Here's how the part is built. I have some questions about the finished solid (model axes, mm). Round coordinates to 2 decimals unless told otherwise and drop trailing zeros. Write each loop counter-clockwise with the first axis right and the second up, starting at its lowest first coordinate (ties: lowest second). Pieces come first, ordered by that corner, then holes. Notation, with made-up numbers: (74.25, 34.25) - (97.25, 34.25) arc R26 ccw to (97.25, 54.25) - close; hole circle Ø4 at (-34, 10). An arc over 180 degrees is marked (long way). One line per item, written item: value. Start each with the question number.
Item 1: Imagine slicing it at B-B, the plane z = 12. Please give me the cut outline in (x, y), then the cut area to 3 significant figures.
Item 2: Imagine slicing it at A-A, the plane y = -17. Please give me the cut outline in (x, z), then the cut area to 3 significant figures.
Item 3: For P1, Ø3, axis at x = 3, z = 19, coming from the +Y side, with a flat end and sliding along its axis, tell me the tip position at first contact or that it passes through.
Item 4: If I drill on line 1 (X direction, y = -3.5, z = 12.75); line 2 (X direction, y = -11.75, z = 1); line 3 (Z direction, x = 18.75, y = -2), over which ranges is the centre line in solid material (lowest first)?
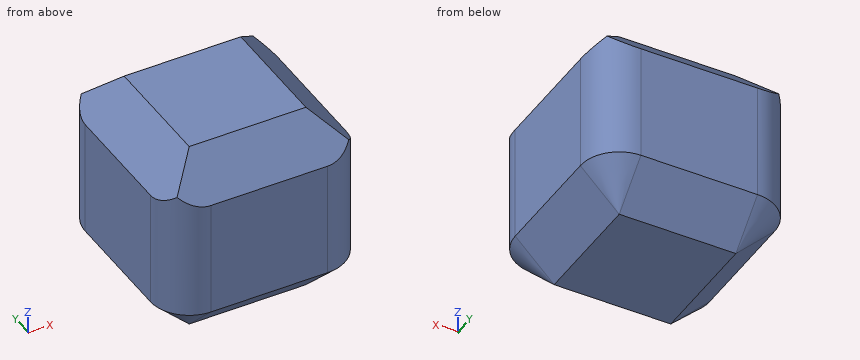
```python
from build123d import *

# Parameters (mm, degrees)
F0_W     = 25.4
F0_H     = 25.4
F1_DEPTH = 25.4
F2_SIZE  = 5.08
F3_R     = 5.08
F4_SIZE  = 5.07999


# Not quite as in the source:
# - a fillet or chamfer is up to 0.001 mm smaller than in the source, because OpenCascade refuses the exact size


with BuildPart() as f1:
    # F0 (on Front) → F1 (new body)
    with BuildSketch(Plane.XZ):
        with Locations((12.7, 12.7)):
            Rectangle(F0_W, F0_H)
    extrude(amount=F1_DEPTH)

    # F2
    f2_edges = [f1.edges().sort_by_distance(p)[0] for p in [
        (25.4, -12.7, 25.4),
        (12.7, -25.4, 25.4),
        (12.7, 0, 25.4),
        (0, -12.7, 25.4),
    ]]
    chamfer(f2_edges, length=F2_SIZE)

    # F3
    f3_edges = [f1.edges().sort_by_distance(p)[0] for p in [
        (25.4, -25.4, 10.16),
        (25.4, 0, 10.16),
        (0, -25.4, 10.16),
        (0, 0, 10.16),
    ]]
    fillet(f3_edges, radius=F3_R)

    # F4 (size 5.08 in the source; OpenCascade refuses exactly that, so slightly less here)
    f4_edges = [f1.edges().sort_by_distance(p)[0] for p in [
        (12.7, -25.4, 0),
    ]]
    chamfer(f4_edges, length=F4_SIZE)


solid = f1.part
```
Values follow:
1. outline: (0, -20.32) arc R5.08 ccw to (5.08, -25.4) - (20.32, -25.4) arc R5.08 ccw to (25.4, -20.32) - (25.4, -5.08) arc R5.08 ccw to (20.32, 0) - (5.08, 0) arc R5.08 ccw to (0, -5.08) - close
1. area: 623 mm^2
2. outline: (0, 5.08) - (5.08, 0) - (20.32, 0) - (25.4, 5.08) - (25.4, 20.32) - (20.32, 25.4) - (5.08, 25.4) - (0, 20.32) - close
2. area: 594 mm^2
3. P1: stops at y = -0.03
4. line 1: x = 0.25 to 25.15
4. line 2: x = 4.08 to 21.32
4. line 3: z = 3.08 to 22.32
